from build123d import *

# Parameters (mm, degrees)
SKETCH1_W           = 152
SKETCH1_H           = 12
BOSS_EXTRUDE1_DEPTH = 125
SKETCH3_W           = 10
SKETCH3_H           = 85
BOSS_EXTRUDE2_DEPTH = 152
SKETCH4_W           = 10
SKETCH4_H           = 39
BOSS_EXTRUDE3_DEPTH = 125
BOSS_EXTRUDE4_DEPTH = 38
BOSS_EXTRUDE5_DEPTH = 38
CUT_EXTRUDE1_DEPTH  = 38
CUT_EXTRUDE2_DEPTH  = 38
SKETCH10_R          = 41
SKETCH10_R_2        = 14
BOSS_EXTRUDE6_DEPTH = 13
CUT_EXTRUDE4_DEPTH  = 13
SKETCH13_R          = 29
CUT_EXTRUDE5_DEPTH  = 38
SKETCH14_R          = 41
SKETCH14_R_2        = 11
BOSS_EXTRUDE8_DEPTH = 13
CUT_EXTRUDE6_DEPTH  = 13


with BuildPart() as part:
    # Sketch1 → Boss-Extrude1 (new body)
    with BuildSketch(Plane.XY):
        with Locations((76, 6)):
            Rectangle(SKETCH1_W, SKETCH1_H)
    extrude(amount=BOSS_EXTRUDE1_DEPTH)

    # Sketch3 → Boss-Extrude2 (add)
    with BuildSketch(Plane(origin=(0, 0, 0), x_dir=(0, 0, -1), z_dir=(1, 0, 0))):
        with Locations((-62.5, 54.5)):
            Rectangle(SKETCH3_W, SKETCH3_H)
    extrude(amount=BOSS_EXTRUDE2_DEPTH)

    # Sketch4 → Boss-Extrude3 (add)
    with BuildSketch(Plane.XY):
        with Locations((76, 31.5)):
            Rectangle(SKETCH4_W, SKETCH4_H)
    extrude(amount=BOSS_EXTRUDE3_DEPTH)

    # Sketch5 → Boss-Extrude4 (add)
    with BuildSketch(Plane(origin=(0, 0, 43.5), x_dir=(-1, 0, 0), z_dir=(0, 0, -1))):
        with BuildLine():
            Line((-36.795408432, 53.709899764), (-49.599242435, 53.709899764))
            ThreePointArc((-49.599242435, 53.709899764), (-96.506096654, 45.20380311), (-88, 92.110657329))
            Line((-88, 92.110657329), (-88, 104.914491332))
            ThreePointArc((-88, 104.914491332), (-104.991378029, 36.718521736), (-36.795408432, 53.709899764))
        make_face()
    extrude(amount=-BOSS_EXTRUDE4_DEPTH)

    # Sketch7 → Boss-Extrude5 (add)
    with BuildSketch(Plane(origin=(0, 0, 43.5), x_dir=(-1, 0, 0), z_dir=(0, 0, -1))):
        with BuildLine():
            ThreePointArc((-88, 104.914491332), (-94.245259526, 102.42652413), (-100, 98.951440042))
            Line((-100, 98.951440042), (-100, 118.511414894))
            ThreePointArc((-100, 118.511414894), (-94.107673916, 120.810826665), (-88, 122.454943601))
            Line((-88, 122.454943601), (-88, 104.914491332))
        make_face()
        with BuildLine():
            Line((-23.19848487, 41.709899764), (-42.758459723, 41.709899764))
            ThreePointArc((-42.758459723, 41.709899764), (-39.283375634, 47.464640238), (-36.795408432, 53.709899764))
            Line((-36.795408432, 53.709899764), (-19.254956164, 53.709899764))
            ThreePointArc((-19.254956164, 53.709899764), (-20.899073099, 47.602225848), (-23.19848487, 41.709899764))
        make_face()
    extrude(amount=-BOSS_EXTRUDE5_DEPTH)

    # Sketch8 → Cut-Extrude1 (cut)
    with BuildSketch(Plane(origin=(0, 0, 57.5), x_dir=(-1, 0, 0), z_dir=(0, 0, -1))):
        with BuildLine():
            Line((-152, 12), (-112.808217889, 83.76966432))
            ThreePointArc((-112.808217889, 83.76966432), (-108.334991946, 90.917999571), (-102.493954541, 97))
            Line((-102.493954541, 97), (-152, 97))
            Line((-152, 97), (-152, 12))
        make_face()
    extrude(amount=-CUT_EXTRUDE1_DEPTH, mode=Mode.SUBTRACT)

    # Sketch9 → Cut-Extrude2 (cut)
    with BuildSketch(Plane(origin=(0, 0, 43.5), x_dir=(-1, 0, 0), z_dir=(0, 0, -1))):
        with BuildLine():
            Line((0, 12), (-23.19848487, 41.709899764))
            ThreePointArc((-23.19848487, 41.709899764), (-20.899073099, 47.602225848), (-19.254956164, 53.709899764))
            Line((-19.254956164, 53.709899764), (-49.599242435, 53.709899764))
            ThreePointArc((-49.599242435, 53.709899764), (-58.248729295, 42.777556047), (-71, 37.14418605))
            Line((-71, 37.14418605), (-71, 51))
            Line((-71, 51), (-81, 51))
            Line((-81, 51), (-81, 37.14418605))
            ThreePointArc((-81, 37.14418605), (-104.767659641, 62.046327903), (-88, 92.110657329))
            Line((-88, 92.110657329), (-88, 97))
            Line((-88, 97), (0, 97))
            Line((0, 97), (0, 12))
        make_face()
    extrude(amount=-CUT_EXTRUDE2_DEPTH, mode=Mode.SUBTRACT)

    # Sketch10 → Boss-Extrude6 (add)
    with BuildSketch(Plane(origin=(0, 0, 43.5), x_dir=(-1, 0, 0), z_dir=(0, 0, -1))):
        with Locations((-76, 65.709899764)):
            Circle(SKETCH10_R)
        with Locations((-76, 65.709899764)):
            Circle(SKETCH10_R_2, mode=Mode.SUBTRACT)
    extrude(amount=BOSS_EXTRUDE6_DEPTH)

    # Sketch11 → Cut-Extrude4 (cut)
    with BuildSketch(Plane(origin=(81, 0, 0), x_dir=(0, 0, -1), z_dir=(1, 0, 0))):
        Polygon((-30.5, 25.015919866), (-30.5, 51), (0, 51), (0, 12), (-0.340530313, 11.874434651), align=None)
    extrude(amount=-CUT_EXTRUDE4_DEPTH, mode=Mode.SUBTRACT)

    # Sketch13 → Cut-Extrude5 (cut)
    with BuildSketch(Plane(origin=(0, 0, 43.5), x_dir=(-1, 0, 0), z_dir=(0, 0, -1))):
        with Locations((-76, 65.709899764)):
            Circle(SKETCH13_R)
    extrude(amount=-CUT_EXTRUDE5_DEPTH, mode=Mode.SUBTRACT)

    # Sketch14 → Boss-Extrude8 (add)
    with BuildSketch(Plane.XY.offset(81.5)):
        with Locations((76, 65.709899764)):
            Circle(SKETCH14_R)
        with Locations((76, 65.709899764)):
            Circle(SKETCH14_R_2, mode=Mode.SUBTRACT)
    extrude(amount=BOSS_EXTRUDE8_DEPTH)

    # Sketch15 → Cut-Extrude6 (cut)
    with BuildSketch(Plane.ZY.offset(-71)):
        Polygon((125, 12), (94.5, 25.015919866), (94.5, 51), (125, 51), align=None)
    extrude(amount=-CUT_EXTRUDE6_DEPTH, mode=Mode.SUBTRACT)


solid = part.part
Geometry: final body of the model. Coordinates: model frame, mm. A direction names the side the tool comes from. Coordinates: 2 decimals unless noted, no trailing zeros. Order: outer loops, then holes, each group sorted by start corner. A loop starts at its lowest first (then second) coordinate and runs counter-clockwise, first axis right, second up.
(1) Section query D-D (y = 44). Return the cut outline in (x, z).
(2) Section query B-B (x = 76). Return the cut outline in (y, z), plus the area to 3 significant figures.
(3) First-contact query: pin 1 (12 mm diameter, centred on y = 71.5, z = 37, fed in from -X); pin 2 (6.5 mm diameter, centred on y = 17, z = 17, fed in from +X); pin 3 (6.5 mm diameter, centred on y = 17.5, z = 33, fed in from -X). Flat tips, straight axial feed; report the tip coordinate or a pass-through.
(4) Material intervals for probe 1 along Y at (x, z) = (76, 86.5); probe 2 along Y at (x, z) = (76, 39.75); probe 3 along Z at (x, y) = (74.5, 97), sorted ascending.
(5) Draft query along Z for faces 1 (the face through (33, 41.71, 50)), 2 (the face through (94, 111, 81.5)), 3 (the face through (34, 53.71, 62)). Return one class per face: pulls with the +Z half, pulls with the -Z half, needs draft (parallel to the pull), parting line crosses it, or undercut.
(6) Section query A-A (z = 48.5). Return the cut outline in (x, y), plus the area to 3 significant figures.
(7) Access query for faces 4 (the face through (31, 48, 81.5)), 5 (the face through (85, 57, 94.5)), 6 (the face through (88, 107, 62)), 7 (the face through (31, 48, 43.5)). Directions: +Z, -Z, +X, -X, +Y, -Y. A direction counts if a zero-diameter tool reaches every point of the face in a straight line with its end or side. Return the directions, or none.
(8) Section query C-C (z = 36). Return the cut outline in (x, y), plus the area to 3 significant figures.
Solution:
1. outline: (22.22, 43.5) - (41.22, 43.5) - (41.22, 30.5) - (110.78, 30.5) - (110.78, 57.5) - (134.53, 57.5) - (134.53, 67.5) - (110.78, 67.5) - (110.78, 94.5) - (41.22, 94.5) - (41.22, 81.5) - (22.22, 81.5) - close; hole (56.77, 43.5) - (95.23, 43.5) - (95.23, 81.5) - (56.77, 81.5) - close
2. outline: (0, 0) - (12, 0) - (11.87, 0.34) - (25.02, 30.5) - (51.71, 30.5) - (51.71, 43.5) - (36.71, 43.5) - (36.71, 81.5) - (54.71, 81.5) - (54.71, 94.5) - (25.02, 94.5) - (12, 125) - (0, 125) - close; (76.71, 81.5) - (106.71, 81.5) - (106.71, 94.5) - (76.71, 94.5) - close; (79.71, 30.5) - (106.71, 30.5) - (106.71, 43.5) - (79.71, 43.5) - close
2. area: 4,640 mm2
3. pin 1: stops at x = 35
3. pin 2: stops at x = 81
3. pin 3: stops at x = 71
4. probe 1: y = 0 to 54.71, 76.71 to 106.71
4. probe 2: y = 0 to 51.71, 79.71 to 106.71
4. probe 3: z = 30.5 to 43.5, 81.5 to 94.5
5. face 1: needs draft
5. face 2: pulls with the +Z half
5. face 3: undercut
6. outline: (0, 0) - (152, 0) - (152, 12) - (81, 12) - (81, 25.02) arc R41 ccw to (100, 98.95) - (100, 118.51) arc R58 ccw to (88, 122.45) - (88, 92.11) arc R29 cw (long way) to (49.6, 53.71) - (19.25, 53.71) arc R58 ccw to (23.2, 41.71) - (42.76, 41.71) arc R41 ccw to (71, 25.02) - (71, 12) - (0, 12) - close
6. area: 4,080 mm2
7. face 4: +Z, -X
7. face 5: +Z, +X, -X, +Y
7. face 6: -X, +Y
7. face 7: -Z, -X
8. outline: (0, 0) - (152, 0) - (152, 12) - (81, 12) - (81, 25.02) arc R41 ccw (long way) to (71, 25.02) - (71, 12) - (0, 12) - close; hole circle Ø28 at (76, 65.71)
8. area: 6,620 mm2
